Design review of the part built by this model. Coordinates are the model's own, in mm. A direction names the side the tool comes from. Coordinates: 2 decimals unless noted, no trailing zeros. Loops run counter-clockwise (first coordinate to the right, second up) from the corner with the lowest first, then second, coordinate; pieces in that order, holes last. Notation, with made-up numbers: M 13,-40 L 51,-40 A27 ccw 51,-23 Z; hole C 19,31.5 d7. An arc over 180 degrees is marked long. Answer as a JSON object with one key per item and string values. Group by question number.
1. Insertion check: pin 1 (1 mm diameter, centred on x = -1.5, z = 1, fed in from -Y); pin 2 (2 mm diameter, centred on x = -4, z = 1.5, fed in from +Y). Each pin has a flat end and moves straight along its axis. Give the tip position at first contact, or say it passes through.
2. To check wall thickness, follow probe 1 along X at (y, z) = (0, 1.75); probe 2 along Z at (x, y) = (1.25, 0.75); probe 3 along Z at (x, y) = (2.75, -1.25). State the ranges of each line that lie inside material, in increasing order.
3. Machinability: for faces 5 (the flat face through (3.691, -1, 2)), 6 (the flat face through (1.72, -1.76, -0.72)), which of the approach directions +Z, -Z, +X, -X, +Y, -Y give a long, thin tool a straight path to every point of the face, cutting with its end or side? Answer none if there is none.
4. Consider section A-A (x = -1.5). State the section outline as (y, z) points.
5. Draft analysis for pull direction Z (two halves, no side actions). For faces 1 (the cylindrical face through (-3.768, 3.233, 1.341)), 2 (the flat face through (1.72, -0.74, -1.75)), 3 (the flat face through (-5, 0, 0)), 4 (the flat face through (1.72, 0.74, 1.75)), state which applies: +Z half, -Z half, draft (parallel to the pull), parting line (faces both ways), or undercut.
from build123d import *

# Parameters (mm, degrees)
CUT_EXTRUDE2_DEPTH = 4


with BuildPart() as part:
    # Sketch4 → Revolve4 (revolve)
    with BuildSketch(Plane.XY):
        Polygon((-5, 0), (0, 0), (3.690598923, 0), (3.690598923, 3), (0, 3), (-1.309401077, 3), (-2.5, 3.5), (-5, 3.5), align=None)
    revolve(axis=Axis((0, 0, 0), (-1, 0, 0)))

    # Sketch6 → Cut-Extrude2 (cut)
    with BuildSketch(Plane(origin=(3.690598923, 0, 0), x_dir=(0, 0, -1), z_dir=(1, 0, 0))):
        Polygon((-2.056545181, 0), (-1.454197043, -1.454197043), (0, -2.056545181), (1.454197043, -1.454197043), (2.056545181, 0), (1.454197043, 1.454197043), (0, 2.056545181), (-1.454197043, 1.454197043), align=None)
    extrude(amount=-CUT_EXTRUDE2_DEPTH, mode=Mode.SUBTRACT)


solid = part.part
Findings below:
{
 "1": {"pin 1": "stops at y = -3.17", "pin 2": "stops at y = 3.46"},
 "2": {"probe 1": "x = -5 to -0.31", "probe 2": "z = -2.9 to -1.75, 1.75 to 2.9", "probe 3": "z = -2.73 to -1.54, 1.54 to 2.73"},
 "3": {"face 5": "+Z, -Z, +X, +Y, -Y", "face 6": "+X"},
 "4": {"outline": "C 0,0 d6.16"},
 "5": {"face 1": "parting line", "face 2": "undercut", "face 3": "draft", "face 4": "undercut"}
}
